The drawing under review shows one solid part. Ordinate dimensions are in mm from its lowest x, y, z. A direction names the side the tool comes from. Round coordinates to 2 decimals unless told otherwise and drop trailing zeros. Order: outer loops, then holes, each group sorted by start corner. A loop starts at its lowest first (then second) coordinate and runs counter-clockwise, first axis right, second up. Notation, with made-up numbers: M 69.5,20.5 L 127.5,20.5 A27 cw 127.5,51.5 Z; hole C -30.5,33.25 d3. An arc over 180 degrees is marked long. Use a Markdown table: item, result.
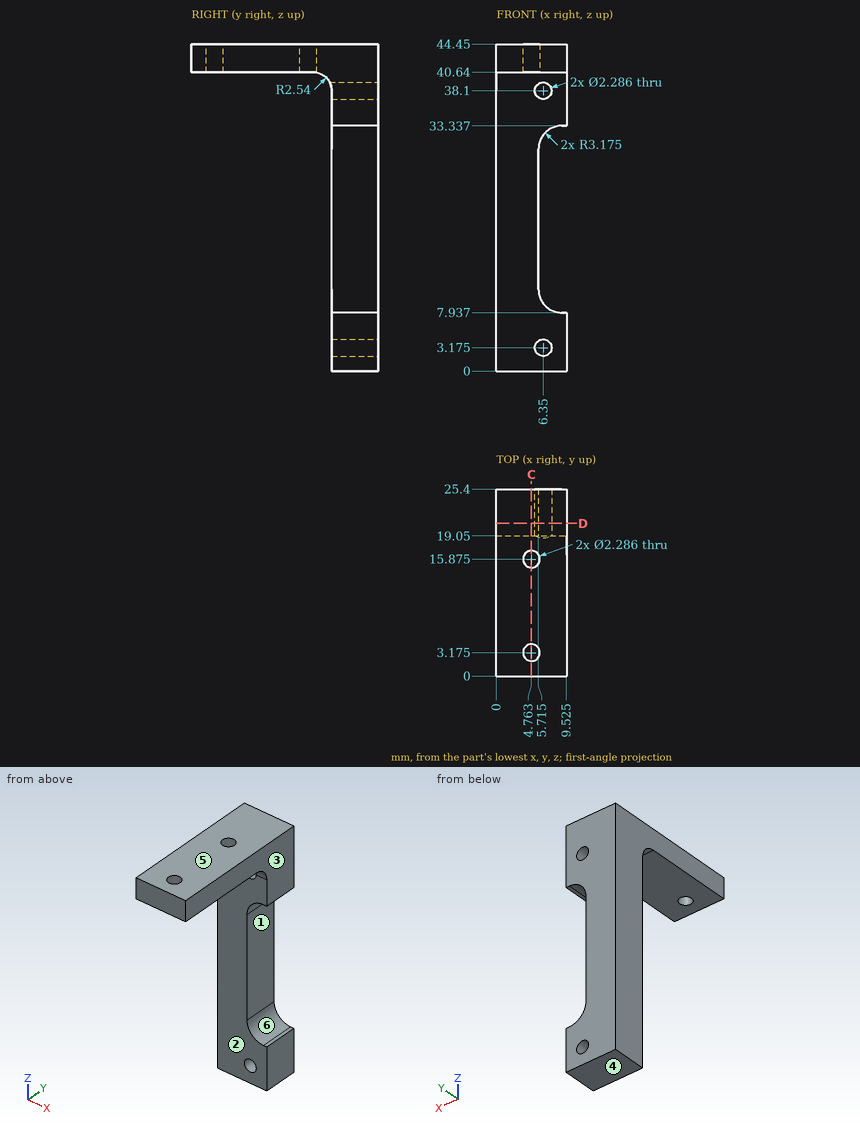
Q1. Machinability: for the marked faces 1, 2 and 3, which of the approach directions +Z, -Z, +X, -X, +Y, -Y give a long, thin tool a straight path to every point of the face, cutting with its end or side? Answer none if there is none.
Determined:
| item | result |
|---|---|
| face 1 | +X, +Y, -Y |
| face 2 | -Z, +X, -X, -Y |
| face 3 | +Z, -Z, +X, +Y, -Y |
Q2. Draft analysis for pull direction Z (two halves, no side actions). For the marked faces 4, 5 and 6, state which applies: pulls with the +Z half, pulls with the -Z half, needs draft (parallel to the pull), parting line crosses it, or undercut.
Determined:
| item | result |
|---|---|
| face 4 | pulls with the -Z half |
| face 5 | pulls with the +Z half |
| face 6 | undercut |
Q3. Wall thickness on line 1 along X through (y, z) = (22.75, 38.1) (1 decimal); line 2 along X through (y, z) = (20.5, 18) (1 decimal); line 3 along Y through (x, z) = (3.5, 20): over which ranges is each line inside the solid? List them lowest first. Write a range as [from, to].
Determined:
| item | result |
|---|---|
| line 1 | x = [0, 5.2], [7.5, 9.5] |
| line 2 | x = [0, 5.7] |
| line 3 | y = [19.05, 25.4] |
Q4. Clearance check with flat-ended pins moving along their axes: pin 1 (3 mm diameter, centred on x = 3, z = 26, fed in from -Y); pin 2 (3 mm diameter, centred on x = 6, z = 14.5, fed in from +Y); pin 3 (1.5 mm diameter, centred on x = 4, y = 16, fed in from -Z); pin 4 (3 mm diameter, centred on y = 22, z = 17.5, fed in from +X) (1 decimal). State where each tip first meets the part, or that it passes through.
Determined:
| item | result |
|---|---|
| pin 1 | stops at y = 19.05 |
| pin 2 | stops at y = 25.4 |
| pin 3 | stops at z = 40.63 |
| pin 4 | stops at x = 5.7 |
Q5. Add section D-D (y = 20.75). Give the number of separate pieces and of enclosed holes in the cut face, then the cut area to 3 significant figures.
Determined:
| item | result |
|---|---|
| separate pieces | 1 |
| enclosed holes | 2 |
| area | 323 mm^2 |
Q6. Add section C-C (x = 4.75). Write out the cut boundary in (y, z).
Determined:
| item | result |
|---|---|
| outline | M 0,40.64 L 2.03,40.64 L 2.03,44.45 L 0,44.45 Z; M 4.32,40.64 L 14.73,40.64 L 14.73,44.45 L 4.32,44.45 Z; M 17.02,40.59 A2.54 cw 19.05,38.1 L 19.05,0 L 25.4,0 L 25.4,44.45 L 17.02,44.45 Z |
